For this review, take the finished solid that the model builds, in its own axes (mm). Face numbers are marked on the shaded views. Give positions to 0.01 mm unless a question says otherwise; leave off trailing zeros. Write each loop counter-clockwise with the first axis right and the second up, starting at its lowest first coordinate (ties: lowest second). Pieces come first, ordered by that corner, then holes.
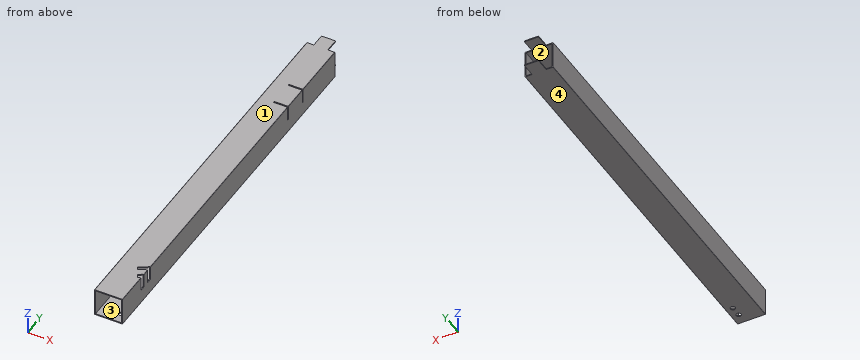
from build123d import *

# Parameters (mm, degrees)
SKETCH1_W           = 37
SKETCH1_H           = 37
BOSS_EXTRUDE1_DEPTH = 571
SKETCH2_W           = 10
SKETCH2_H           = 20
CUT_EXTRUDE1_DEPTH  = 40
SKETCH3_W           = 21
SKETCH3_H           = 2
CUT_EXTRUDE2_DEPTH  = 20
CUT_EXTRUDE3_START  = -40
CUT_EXTRUDE3_DEPTH  = 20
SKETCH5_R           = 3.5
CUT_EXTRUDE4_DEPTH  = 10


with BuildPart() as part:
    # Sketch1 → Boss-Extrude1 (new body)
    with BuildSketch(Plane(origin=(0, 0, 0), x_dir=(1, 0, 0), z_dir=(0, 1, 0))):
        with BuildLine():
            Line((0.5, 0), (39.5, 0))
            ThreePointArc((39.5, 0), (39.853553391, 0.146446609), (40, 0.5))
            Line((40, 0.5), (40, 39.5))
            ThreePointArc((40, 39.5), (39.853553391, 39.853553391), (39.5, 40))
            Line((39.5, 40), (0.5, 40))
            ThreePointArc((0.5, 40), (0.146446609, 39.853553391), (0, 39.5))
            Line((0, 39.5), (0, 0.5))
            ThreePointArc((0, 0.5), (0.146446609, 0.146446609), (0.5, 0))
        make_face()
        with Locations((20, 20)):
            Rectangle(SKETCH1_W, SKETCH1_H, mode=Mode.SUBTRACT)
    extrude(amount=BOSS_EXTRUDE1_DEPTH)

    # Sketch2 → Cut-Extrude1 (cut)
    with BuildSketch(Plane.XY.offset(-40)):
        with Locations((35, 561)):
            Rectangle(SKETCH2_W, SKETCH2_H)
        with Locations((5, 561)):
            Rectangle(SKETCH2_W, SKETCH2_H)
    extrude(amount=CUT_EXTRUDE1_DEPTH, mode=Mode.SUBTRACT)

    # Sketch3 → Cut-Extrude2 (cut)
    with BuildSketch(Plane(origin=(40, 0, 0), x_dir=(0, 0, -1), z_dir=(1, 0, 0))):
        with Locations((10.5, 467.5)):
            Rectangle(SKETCH3_W, SKETCH3_H)
        with Locations((10.5, 429.5)):
            Rectangle(SKETCH3_W, SKETCH3_H)
    extrude(amount=-CUT_EXTRUDE2_DEPTH, mode=Mode.SUBTRACT)

    # Sketch4 → Cut-Extrude3 (cut)
    with BuildSketch(Plane(origin=(0, 0, -40), x_dir=(-1, 0, 0), z_dir=(0, 0, -1)).offset(CUT_EXTRUDE3_START)):
        Polygon((-40, 72.59987752), (-37, 72.59987752), (-37, 70.867826713), (-25.659711467, 64.320508076), (-28.159711467, 59.990381057), (-37, 65.094324021), (-40, 65.094324021), align=None)
        Polygon((-40, 55.279369445), (-37, 55.279369445), (-37, 53.547318637), (-33.159711467, 51.330127019), (-35.659711467, 47), (-37, 47.773815945), (-40, 47.773815945), align=None)
    extrude(amount=CUT_EXTRUDE3_DEPTH, mode=Mode.SUBTRACT)

    # Sketch5 → Cut-Extrude4 (cut)
    with BuildSketch(Plane(origin=(0, 0, -40), x_dir=(-1, 0, 0), z_dir=(0, 0, -1))):
        with Locations((-30, 15)):
            Circle(SKETCH5_R)
        with Locations((-30, 30)):
            Circle(SKETCH5_R)
    extrude(amount=-CUT_EXTRUDE4_DEPTH, mode=Mode.SUBTRACT)


solid = part.part
(1) We need section A-A (z = -13.5). Write out the cut boundary in (x, y), and give its area (3 significant figures).
(2) Clearance check with flat-ended pins moving along their axes: pin 1 Ø1.2 at (y, z) = (559, -39.5) entering from +X; pin 2 Ø1.2 at (y, z) = (468, -0.5) entering from +X; pin 3 Ø0.8 at (y, z) = (71.5, -0.5) entering from +X; pin 4 Ø1.5 at (x, z) = (38.5, -14.5) entering from +Y. State where each tip first meets the part, or that it passes through.
(3) The part is to be moulded in two halves that separate along Z. For the marked faces 1, 2, 3 and 4, say which applies: +Z half, -Z half, draft (parallel to the pull), parting line (faces both ways), or undercut.
(4) We need section B-B (y = 412.5). Write out the cut boundary in (x, z), and give its area (3 significant figures).
(5) For L1, parallel to Z at x = 12, y = 426.5; L2, parallel to X at y = 507, z = -10, list the stretches that pass through material, from the lowest coordinate up.
The answers:
1. outline: (0, 0) - (1.5, 0) - (1.5, 551) - (0, 551) - close; (38.5, 0) - (40, 0) - (40, 47.77) - (38.5, 47.77) - close; (38.5, 55.28) - (40, 55.28) - (40, 65.09) - (38.5, 65.09) - close; (38.5, 72.6) - (40, 72.6) - (40, 428.5) - (38.5, 428.5) - close; (38.5, 430.5) - (40, 430.5) - (40, 466.5) - (38.5, 466.5) - close; (38.5, 468.5) - (40, 468.5) - (40, 551) - (38.5, 551) - close
1. area: 1,620 mm2
2. pin 1: stops at x = 30
2. pin 2: stops at x = 40
2. pin 3: stops at x = 37
2. pin 4: stops at y = 551
3. face 1: +Z half
3. face 2: undercut
3. face 3: undercut
3. face 4: -Z half
4. outline: (0, -39.5) arc R0.5 ccw to (0.5, -40) - (39.5, -40) arc R0.5 ccw to (40, -39.5) - (40, -0.5) arc R0.5 ccw to (39.5, 0) - (0.5, 0) arc R0.5 ccw to (0, -0.5) - close; hole (1.5, -38.5) - (38.5, -38.5) - (38.5, -1.5) - (1.5, -1.5) - close
4. area: 231 mm2
5. L1: z = -40 to -38.5, -1.5 to 0
5. L2: x = 0 to 1.5, 38.5 to 40
